Verification items for the finished model (mm, model axes). Face numbers are marked on the shaded views. A direction names the side the tool comes from. Round coordinates to 2 decimals unless told otherwise and drop trailing zeros. Write each loop counter-clockwise with the first axis right and the second up, starting at its lowest first coordinate (ties: lowest second). Pieces come first, ordered by that corner, then holes.
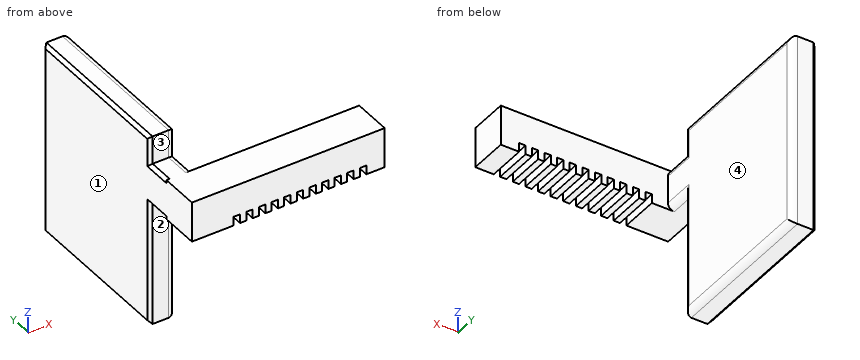
from build123d import *

# Parameters (mm, degrees)
SKETCH2_W           = 60
SKETCH2_H           = 50
BOSS_EXTRUDE1_DEPTH = 4
SKETCH3_W           = 8
SKETCH3_H           = 12.5
BOSS_EXTRUDE2_DEPTH = 20
FILLET2_R           = 2
CHAMFER2_SIZE       = 1
SKETCH4_W           = 60
SKETCH4_H           = 12.5
BOSS_EXTRUDE4_DEPTH = 12
SKETCH10_W          = 2
SKETCH10_H          = 2.8
CUT_EXTRUDE1_DEPTH  = 87.02325267
LPATTERN5_COUNT     = 11
LPATTERN5_PITCH     = 3.927


with BuildPart() as part:
    # Sketch2 → Boss-Extrude1 (new, symmetric)
    with BuildSketch(Plane(origin=(0, 0, 0), x_dir=(0, 0, -1), z_dir=(1, 0, 0))):
        Rectangle(SKETCH2_W, SKETCH2_H)
    extrude(amount=BOSS_EXTRUDE1_DEPTH, both=True)

    # Sketch3 → Boss-Extrude2 (add)
    with BuildSketch(Plane.XZ.offset(25)):
        with Locations((0, 15)):
            Rectangle(SKETCH3_W, SKETCH3_H)
    extrude(amount=BOSS_EXTRUDE2_DEPTH)

    # Fillet2
    fillet2_edges = [part.edges().sort_by_distance(p)[0] for p in [
        (4, 0, 30),
        (4, -25, -10.625),
        (4, -25, 25.625),
        (4, -35, 8.75),
        (4, -35, 21.25),
        (4, -45, 15),
        (4, 0, -30),
        (4, 25, 0),
    ]]
    fillet(fillet2_edges, radius=FILLET2_R)

    # Chamfer2
    chamfer2_edges = [part.edges().sort_by_distance(p)[0] for p in [
        (-4, -25, -10.625),
        (-4, -35, 21.25),
        (-4, -35, 8.75),
        (-4, -45, 15),
        (-4, -25, 25.625),
        (-4, 0, 30),
        (-4, 25, 0),
        (-4, 0, -30),
    ]]
    chamfer(chamfer2_edges, length=CHAMFER2_SIZE)

    # Sketch4 → Boss-Extrude4 (add)
    with BuildSketch(Plane.XZ.offset(45)):
        with Locations((26, 15)):
            Rectangle(SKETCH4_W, SKETCH4_H)
    extrude(amount=-BOSS_EXTRUDE4_DEPTH)

    # Sketch10 → Cut-Extrude1 (cut, symmetric)
    with BuildSketch(Plane(origin=(0, -33, 0), x_dir=(1, 0, 0), z_dir=(0, 1, 0))):
        with Locations((10, -10.15)):
            Rectangle(SKETCH10_W, SKETCH10_H)
    cut_extrude1 = extrude(amount=CUT_EXTRUDE1_DEPTH, both=True, mode=Mode.SUBTRACT)

    # LPattern5: Cut-Extrude1 ×11
    with Locations(*[(i * LPATTERN5_PITCH, 0, 0) for i in range(1, LPATTERN5_COUNT)]):
        add(cut_extrude1, mode=Mode.SUBTRACT)


solid = part.part
Q1. Sectioned sample at B-B (y = -12). Enter the section's corners in (x, z).
Recorded:
outline: (-4, -29) - (-3, -30) - (2, -30) arc R2 ccw to (4, -28) - (4, 28) arc R2 ccw to (2, 30) - (-3, 30) - (-4, 29) - close
Q2. Sectioned sample at C-C (x = 12). Enter the section's corners in (y, z).
Recorded:
outline: (-45, 8.75) - (-33, 8.75) - (-33, 21.25) - (-45, 21.25) - close
Q3. Sectioned sample at A-A (z = 7). Enter the section's corners in (x, y).
Recorded:
outline: (-4, -24) - (-3, -25) - (2, -25) arc R2 ccw to (4, -23) - (4, 23) arc R2 ccw to (2, 25) - (-3, 25) - (-4, 24) - close
Q4. Material ranges on line 1 along X through (y, z) = (20.5, -19); line 2 along Y through (x, z) = (5, 18); line 3 along Z through (x, y) = (5.5, -33.5), recorded low to high.
Recorded:
line 1: x = -4 to 4
line 2: y = -45 to -33
line 3: z = 8.75 to 21.25
Q5. Depth check by flat-ended pin: P1, Ø12, axis at x = 23.5, z = 17.5, coming from the +Y side; P2, Ø0.6, axis at x = 19.5, y = -37.5, coming from the -Z side; P3, Ø12, axis at y = -1.5, z = 7.5, coming from the +X side. Enter the tip coordinate at first touch or a pass-through.
Recorded:
P1: stops at y = -33
P2: stops at z = 8.75
P3: stops at x = 4
Q6. Tool access check on the marked faces 1, 2, 3 and 4. Record the directions out of +Z, -Z, +X, -X, +Y, -Y that give a thin tool (end or side, any length) a straight path to the whole face; none if there is none.
Recorded:
face 1: +Z, -Z, -X, +Y, -Y
face 2: -Z, +X, -X, -Y
face 3: +Z, +X, -X, -Y
face 4: +Z, -Z, +X, +Y
